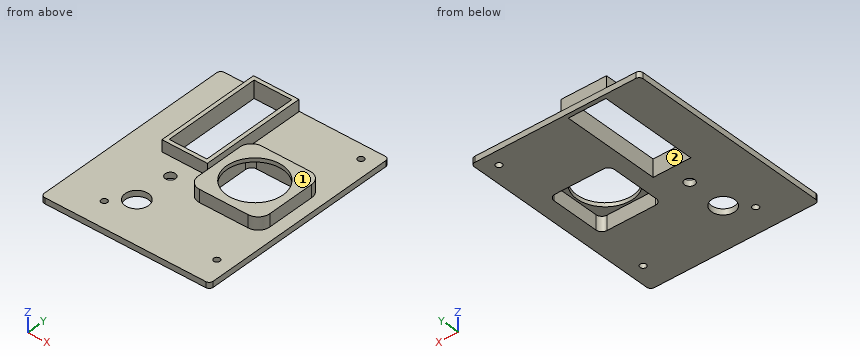
from build123d import *

# Parameters (mm, degrees)
IZIM1_W                 = 87
IZIM1_H                 = 107
TAPA_DEPTH              = 3
REDONDEO1_R             = 2
IZIM3_R                 = 1.6
HUECOSPLACA_DEPTH       = 3
IZIM2_R                 = 1.6
HUECODISIPADOR_DEPTH    = 3
HUECOFAN_DEPTH          = 10
SALIENTE_EXTRUIR4_START = 4.5
SALIENTE_EXTRUIR4_DEPTH = 4.5
SALIENTE_EXTRUIR5_START = -3
CROQUIS8_W              = 37.30700553
CROQUIS8_H              = 38.753013496
SALIENTE_EXTRUIR5_DEPTH = 3
SALIENTE_EXTRUIR6_START = 2
CROQUIS9_R              = 14.5
SALIENTE_EXTRUIR6_DEPTH = 2
CROQUIS10_R             = 2.6
CROQUIS10_R_2           = 6
LEDANDBUZZER_DEPTH      = 10
CROQUIS11_W             = 19.4
CROQUIS11_H             = 50.6
DISPLAY_DEPTH           = 10
CROQUIS12_W             = 23.4
CROQUIS12_H             = 54.6
CROQUIS12_W_2           = 19.4
CROQUIS12_H_2           = 50.6
SALIENTE_EXTRUIR7_DEPTH = 6


with BuildPart() as part:
    # Çizim1 → Tapa (new body)
    with BuildSketch(Plane.XY):
        Rectangle(IZIM1_W, IZIM1_H)
    extrude(amount=TAPA_DEPTH)

    # Redondeo1
    redondeo1_edges = [part.edges().sort_by_distance(p)[0] for p in [
        (43.5, -53.5, 1.5),
        (-43.5, -53.5, 1.5),
        (-43.5, 53.5, 1.5),
        (43.5, 53.5, 1.5),
    ]]
    fillet(redondeo1_edges, radius=REDONDEO1_R)

    # Çizim3 → HuecosPlaca (cut)
    with BuildSketch(Plane.XY.offset(3)):
        with Locations((35.5, 46)):
            Circle(IZIM3_R)
        with Locations((35.5, -40)):
            Circle(IZIM3_R)
        with Locations(Location((-22.5, 46, 0), (0, 0, 180))):
            Circle(IZIM3_R)
        with Locations(Location((-22.5, -40, 0), (0, 0, 180))):
            Circle(IZIM3_R)
    extrude(amount=-HUECOSPLACA_DEPTH, mode=Mode.SUBTRACT)

    # Çizim2 → HuecoDisipador (cut)
    with BuildSketch(Plane.XY.offset(3)):
        with Locations((34.8, 18)):
            Circle(IZIM2_R)
        with Locations((34.8, -14)):
            Circle(IZIM2_R)
        with Locations(Location((2.8, -14, 0), (0, 0, 180))):
            Circle(IZIM2_R)
        with Locations(Location((2.8, 18, 0), (0, 0, 180))):
            Circle(IZIM2_R)
    extrude(amount=-HUECODISIPADOR_DEPTH, mode=Mode.SUBTRACT)

    # Croquis1 → HuecoFan (cut)
    with BuildSketch(Plane.XY.offset(3)):
        with BuildLine():
            Line((6.3, -13.5), (31.3, -13.5))
            ThreePointArc((31.3, -13.5), (33.421320344, -12.621320344), (34.3, -10.5))
            Line((34.3, -10.5), (34.3, 14.5))
            ThreePointArc((34.3, 14.5), (33.421320344, 16.621320344), (31.3, 17.5))
            Line((31.3, 17.5), (6.3, 17.5))
            ThreePointArc((6.3, 17.5), (4.178679656, 16.621320344), (3.3, 14.5))
            Line((3.3, 14.5), (3.3, -10.5))
            ThreePointArc((3.3, -10.5), (4.178679656, -12.621320344), (6.3, -13.5))
        make_face()
    extrude(amount=-HUECOFAN_DEPTH, mode=Mode.SUBTRACT)

    # Croquis7 → Saliente-Extruir4 (add)
    with BuildSketch(Plane.XY.offset(3).offset(SALIENTE_EXTRUIR4_START)):
        with BuildLine():
            Line((6.3, -16.5), (31.3, -16.5))
            ThreePointArc((31.3, -16.5), (35.542640687, -14.742640687), (37.3, -10.5))
            Line((37.3, -10.5), (37.3, 14.5))
            ThreePointArc((37.3, 14.5), (35.542640687, 18.742640687), (31.3, 20.5))
            Line((31.3, 20.5), (6.3, 20.5))
            ThreePointArc((6.3, 20.5), (2.057359313, 18.742640687), (0.3, 14.5))
            Line((0.3, 14.5), (0.3, -10.5))
            ThreePointArc((0.3, -10.5), (2.057359313, -14.742640687), (6.3, -16.5))
        make_face()
        with BuildLine():
            Line((6.3, -13.5), (31.3, -13.5))
            ThreePointArc((31.3, -13.5), (33.421320344, -12.621320344), (34.3, -10.5))
            Line((34.3, -10.5), (34.3, 14.5))
            ThreePointArc((34.3, 14.5), (33.421320344, 16.621320344), (31.3, 17.5))
            Line((31.3, 17.5), (6.3, 17.5))
            ThreePointArc((6.3, 17.5), (4.178679656, 16.621320344), (3.3, 14.5))
            Line((3.3, 14.5), (3.3, -10.5))
            ThreePointArc((3.3, -10.5), (4.178679656, -12.621320344), (6.3, -13.5))
        make_face(mode=Mode.SUBTRACT)
    extrude(amount=-SALIENTE_EXTRUIR4_DEPTH)

    # Croquis8 → Saliente-Extruir5 (add)
    with BuildSketch(Plane(origin=(0, 0, 0), x_dir=(-1, 0, 0), z_dir=(0, 0, -1)).offset(SALIENTE_EXTRUIR5_START)):
        with Locations((-18.653502765, 2.530513941)):
            Rectangle(CROQUIS8_W, CROQUIS8_H)
        with BuildLine():
            Line((-3.3, -10.5), (-3.3, 14.5))
            ThreePointArc((-3.3, 14.5), (-4.178679656, 16.621320344), (-6.3, 17.5))
            Line((-6.3, 17.5), (-31.3, 17.5))
            ThreePointArc((-31.3, 17.5), (-33.421320344, 16.621320344), (-34.3, 14.5))
            Line((-34.3, 14.5), (-34.3, -10.5))
            ThreePointArc((-34.3, -10.5), (-33.421320344, -12.621320344), (-31.3, -13.5))
            Line((-31.3, -13.5), (-6.3, -13.5))
            ThreePointArc((-6.3, -13.5), (-4.178679656, -12.621320344), (-3.3, -10.5))
        make_face(mode=Mode.SUBTRACT)
    extrude(amount=SALIENTE_EXTRUIR5_DEPTH)

    # Croquis9 → Saliente-Extruir6 (add)
    with BuildSketch(Plane.XY.offset(7.5).offset(SALIENTE_EXTRUIR6_START)):
        with BuildLine():
            Line((6.3, -16.5), (31.3, -16.5))
            ThreePointArc((31.3, -16.5), (35.542640687, -14.742640687), (37.3, -10.5))
            Line((37.3, -10.5), (37.3, 14.5))
            ThreePointArc((37.3, 14.5), (35.542640687, 18.742640687), (31.3, 20.5))
            Line((31.3, 20.5), (6.3, 20.5))
            ThreePointArc((6.3, 20.5), (2.057359313, 18.742640687), (0.3, 14.5))
            Line((0.3, 14.5), (0.3, -10.5))
            ThreePointArc((0.3, -10.5), (2.057359313, -14.742640687), (6.3, -16.5))
        make_face()
        with Locations((18.8, 2)):
            Circle(CROQUIS9_R, mode=Mode.SUBTRACT)
    extrude(amount=-SALIENTE_EXTRUIR6_DEPTH)

    # Croquis10 → LEDandBUZZER (cut)
    with BuildSketch(Plane.XY.offset(3)):
        with Locations((-13.5, -11)):
            Circle(CROQUIS10_R)
        with Locations((-13.5, -31)):
            Circle(CROQUIS10_R_2)
    extrude(amount=-LEDANDBUZZER_DEPTH, mode=Mode.SUBTRACT)

    # Croquis11 → DISPLAY (cut)
    with BuildSketch(Plane.XY.offset(3)):
        with Locations((-14.5, 26)):
            Rectangle(CROQUIS11_W, CROQUIS11_H)
    extrude(amount=-DISPLAY_DEPTH, mode=Mode.SUBTRACT)

    # Croquis12 → Saliente-Extruir7 (add)
    with BuildSketch(Plane.XY.offset(3)):
        with Locations((-14.5, 26)):
            Rectangle(CROQUIS12_W, CROQUIS12_H)
        with Locations((-14.5, 26)):
            Rectangle(CROQUIS12_W_2, CROQUIS12_H_2, mode=Mode.SUBTRACT)
    extrude(amount=SALIENTE_EXTRUIR7_DEPTH)


solid = part.part
Part model, mm, in its own coordinate system. Face numbers are marked on the shaded views. Give positions to 0.01 mm unless a question says otherwise; leave off trailing zeros. Loops run counter-clockwise (first coordinate to the right, second up) from the corner with the lowest first, then second, coordinate; pieces in that order, holes last.
(1) Drill centre lines: line 1 along X through (y, z) = (6, 4.25); line 2 along Y through (x, z) = (35.5, 0.7); line 3 along Y through (x, z) = (-9, 0.5). Where is each one in solid material? Low to high.
Return value:
line 1: x = -26.2 to -24.2, -4.8 to -2.8, 0.3 to 3.3, 34.3 to 37.3
line 2: y = -53.5 to -41.6, -38.4 to 44.4, 47.6 to 53.5
line 3: y = -53.5 to -34.97, -27.03 to 0.7, 51.3 to 53.5
(2) Band-saw the part on D-D (x = -22.5). Write the cut outline in (y, z).
Return value:
outline: (-53.5, 0) - (-41.6, 0) - (-41.6, 3) - (-53.5, 3) - close; (-38.4, 0) - (0.7, 0) - (0.7, 9) - (-1.3, 9) - (-1.3, 3) - (-38.4, 3) - close; (51.3, 0) - (53.5, 0) - (53.5, 3) - (53.3, 3) - (53.3, 9) - (51.3, 9) - close
(3) Pull direction X, two halves, no side cores. Call the marked faces 1 and 2: pulls with the +X half, pulls with the -X half, needs draft (parallel to the pull), parting line crosses it, or undercut.
Return value:
face 1: needs draft
face 2: undercut
(4) Pin check, flat tips, straight feed: pin 1 (1.8 mm diameter, centred on x = -9.5, z = 4.5, fed in from -Y); pin 2 (18.5 mm diameter, centred on x = -10.5, y = 27, fed in from +Z); pin 3 (4 mm diameter, centred on y = 39, z = 5.5, fed in from -X). Stop position of each tip, or through.
Return value:
pin 1: stops at y = -1.3
pin 2: stops at z = 9
pin 3: stops at x = -26.2
(5) Band-saw the part on B-B (x = -6). Write the cut outline in (y, z), and give its area (3 significant figures).
Return value:
outline: (-53.5, 0) - (0.7, 0) - (0.7, 9) - (-1.3, 9) - (-1.3, 3) - (-53.5, 3) - close; (51.3, 0) - (53.5, 0) - (53.5, 3) - (53.3, 3) - (53.3, 9) - (51.3, 9) - close
area: 193 mm2
(6) Band-saw the part on A-A (y = 46). Write the cut outline in (x, z), and give its area (3 significant figures).
Return value:
outline: (-43.5, 0) - (-24.2, 0) - (-24.2, 9) - (-26.2, 9) - (-26.2, 3) - (-43.5, 3) - close; (-4.8, 0) - (33.9, 0) - (33.9, 3) - (-2.8, 3) - (-2.8, 9) - (-4.8, 9) - close; (37.1, 0) - (43.5, 0) - (43.5, 3) - (37.1, 3) - close
area: 217 mm2
(7) Band-saw the part on C-C (z = 6.25). Write the cut outline in (x, y), and give its area (3 significant figures).
Return value:
outline: (-26.2, -1.3) - (-2.8, -1.3) - (-2.8, 53.3) - (-26.2, 53.3) - close; (0.3, -10.5) arc R6 ccw to (6.3, -16.5) - (31.3, -16.5) arc R6 ccw to (37.3, -10.5) - (37.3, 14.5) arc R6 ccw to (31.3, 20.5) - (6.3, 20.5) arc R6 ccw to (0.3, 14.5) - close; hole (-24.2, 0.7) - (-4.8, 0.7) - (-4.8, 51.3) - (-24.2, 51.3) - close; hole (3.3, -10.5) arc R3 ccw to (6.3, -13.5) - (31.3, -13.5) arc R3 ccw to (34.3, -10.5) - (34.3, 14.5) arc R3 ccw to (31.3, 17.5) - (6.3, 17.5) arc R3 ccw to (3.3, 14.5) - close
area: 681 mm2
